For this review, take the finished solid that the model builds, in its own axes (mm). Round coordinates to 2 decimals unless told otherwise and drop trailing zeros. Loops run counter-clockwise (first coordinate to the right, second up) from the corner with the lowest first, then second, coordinate; pieces in that order, holes last. Notation, with made-up numbers: (34, 15.5) -> (88, 15.5) arc R10 cw to (88, 34.5) -> close; hole circle Ø11 at (10, 19). An arc over 180 degrees is marked (long way). Use one line per item in the form item = value. Start each with the question number.
from build123d import *

# Parameters (mm, degrees)
SKETCH_1_R          = 1.25
SKETCH_1_R_2        = 6.55
EXTRUDE_1_DEPTH     = 1.5
EXTRUDE_2_DEPTH     = 3
SKETCH_3_R          = 0.6
CUT_EXTRUDE_1_DEPTH = 4
SKETCH_4_R          = 1.55
CUT_EXTRUDE_2_DEPTH = 4
CUT_EXTRUDE_3_DEPTH = 4
FILLET_1_R          = 1
CHAMFER_1_SIZE      = 1
SKETCH_6_R          = 1.55
EXTRUDE_3_DEPTH     = 3
CUT_EXTRUDE_4_DEPTH = 4
FILLET_2_R          = 0.6


with BuildPart() as part:
    # 草图1 → 凸台-拉伸1 (new body, symmetric)
    with BuildSketch(Plane.XY):
        with BuildLine():
            Line((-34.52642222, 8.609923977), (-26.496675247, -8.609923977))
            Line((-26.496675247, -8.609923977), (26.496675247, -8.609923977))
            Line((26.496675247, -8.609923977), (34.52642222, 8.609923977))
            Line((34.52642222, 8.609923977), (5.071419141, 22.345017483))
            ThreePointArc((5.071419141, 22.345017483), (0, 23.469324039), (-5.071419141, 22.345017483))
            Line((-5.071419141, 22.345017483), (-34.52642222, 8.609923977))
        make_face()
        with Locations((0, 20.969324039)):
            Circle(SKETCH_1_R, mode=Mode.SUBTRACT)
        with Locations((8.227241336, 6.719324039)):
            Circle(SKETCH_1_R, mode=Mode.SUBTRACT)
        with Locations((-8.227241336, 6.719324039)):
            Circle(SKETCH_1_R, mode=Mode.SUBTRACT)
        with Locations((0, 11.469324039)):
            Circle(SKETCH_1_R_2, mode=Mode.SUBTRACT)
    extrude(amount=EXTRUDE_1_DEPTH, both=True)

    # 草图2 → 凸台-拉伸2 (add)
    with BuildSketch(Plane.XY.offset(1.5)):
        Polygon((-33.258567434, 5.891000616), (-38.696414157, 3.355291045), (-33.202376754, -8.426710186), (-27.764530032, -5.891000616), (-29.032384817, -3.172077255), (-31.705992789, -4.418801127), (-34.664320621, 1.925353382), (-31.990712649, 3.172077255), align=None)
        Polygon((38.696414157, 3.355291045), (33.202376754, -8.426710186), (27.764530032, -5.891000616), (29.032384817, -3.172077255), (31.705992789, -4.418801127), (34.664320621, 1.925353382), (31.990712649, 3.172077255), (33.258567434, 5.891000616), align=None)
    extrude(amount=-EXTRUDE_2_DEPTH)

    # 草图3 → 切除-拉伸1 (cut, through all)
    with BuildSketch(Plane.XY.offset(1.5)):
        with Locations((-33.512138391, 6.434785288)):
            Circle(SKETCH_3_R)
        with Locations((-34.410749664, 1.38156871)):
            Circle(SKETCH_3_R)
        with Locations((-31.959563746, -3.875016455)):
            Circle(SKETCH_3_R)
        with Locations((-29.285955774, -2.628292582)):
            Circle(SKETCH_3_R)
        with Locations((-31.737141692, 2.628292582)):
            Circle(SKETCH_3_R)
        with Locations((-27.510959075, -6.434785288)):
            Circle(SKETCH_3_R)
        with Locations((27.510959075, -6.434785288)):
            Circle(SKETCH_3_R)
        with Locations((31.737141692, 2.628292582)):
            Circle(SKETCH_3_R)
        with Locations((29.285955774, -2.628292582)):
            Circle(SKETCH_3_R)
        with Locations((31.959563746, -3.875016455)):
            Circle(SKETCH_3_R)
        with Locations((34.410749664, 1.38156871)):
            Circle(SKETCH_3_R)
        with Locations((33.512138391, 6.434785288)):
            Circle(SKETCH_3_R)
    extrude(amount=-CUT_EXTRUDE_1_DEPTH, mode=Mode.SUBTRACT)

    # 草图4 → 切除-拉伸2 (cut, through all)
    with BuildSketch(Plane.XY.offset(1.5)):
        with Locations((-29.875181049, 6.917010638)):
            Circle(SKETCH_4_R)
        with Locations((-24.803761908, -3.958682806)):
            Circle(SKETCH_4_R)
        with Locations((24.803761908, -3.958682806)):
            Circle(SKETCH_4_R)
        with Locations((29.875181049, 6.917010638)):
            Circle(SKETCH_4_R)
    extrude(amount=-CUT_EXTRUDE_2_DEPTH, mode=Mode.SUBTRACT)

    # 草图5 → 切除-拉伸3 (cut, through all)
    with BuildSketch(Plane.XY.offset(1.5)):
        with BuildLine():
            Line((-11.487209375, 14.939773688), (-26.491794663, 7.943020661))
            Line((-26.491794663, 7.943020661), (-21.50545883, -2.750211042))
            Line((-21.50545883, -2.750211042), (-10.562941581, 5.775093172))
            ThreePointArc((-10.562941581, 5.775093172), (-11.939435981, 10.265219199), (-11.487209375, 14.939773688))
        make_face()
        with BuildLine():
            Line((-17.384057406, -4.609923977), (-2, -4.609923977))
            Line((-2, -4.609923977), (-2, -0.362835527))
            ThreePointArc((-2, -0.362835527), (-5.267782675, 0.687373117), (-8.104582376, 2.619705713))
            Line((-8.104582376, 2.619705713), (-17.384057406, -4.609923977))
        make_face()
        with BuildLine():
            Line((17.384057406, -4.609923977), (8.104582376, 2.619705713))
            ThreePointArc((8.104582376, 2.619705713), (5.267782675, 0.687373117), (2, -0.362835527))
            Line((2, -0.362835527), (2, -4.609923977))
            Line((2, -4.609923977), (17.384057406, -4.609923977))
        make_face()
        with BuildLine():
            Line((21.50545883, -2.750211042), (10.562941581, 5.775093172))
            ThreePointArc((10.562941581, 5.775093172), (11.939435981, 10.265219199), (11.487209375, 14.939773688))
            Line((11.487209375, 14.939773688), (26.491794663, 7.943020661))
            Line((26.491794663, 7.943020661), (21.50545883, -2.750211042))
        make_face()
    extrude(amount=-CUT_EXTRUDE_3_DEPTH, mode=Mode.SUBTRACT)

    # 圆角1
    fillet_1_edges = [part.edges().sort_by_distance(p)[0] for p in [
        (-2, -0.362835527, 0),
        (-2, -4.609923977, 0),
        (-17.384057406, -4.609923977, 0),
        (-8.104582376, 2.619705713, 0),
        (17.384057406, -4.609923977, 0),
        (2, -4.609923977, 0),
        (2, -0.362835527, 0),
        (8.104582376, 2.619705713, 0),
        (10.562941581, 5.775093172, 0),
        (11.487209375, 14.939773688, 0),
        (26.491794663, 7.943020661, 0),
        (21.50545883, -2.750211042, 0),
        (-21.50545883, -2.750211042, 0),
        (-26.491794663, 7.943020661, 0),
        (-11.487209375, 14.939773688, 0),
        (-10.562941581, 5.775093172, 0),
    ]]
    fillet(fillet_1_edges, radius=FILLET_1_R)

    # 倒角1
    chamfer_1_edges = [part.edges().sort_by_distance(p)[0] for p in [
        (-33.202376754, -8.426710186, 0),
        (-38.696414157, 3.355291045, 0),
        (38.696414157, 3.355291045, 0),
        (33.202376754, -8.426710186, 0),
    ]]
    chamfer(chamfer_1_edges, length=CHAMFER_1_SIZE)

    # 草图6 → 凸台-拉伸3 (add)
    with BuildSketch(Plane.XY.offset(1.5)):
        with BuildLine():
            Line((-11.457456133, 28.190053348), (-20.630385749, 15.089752201))
            Line((-20.630385749, 15.089752201), (-5.071419141, 22.345017483))
            ThreePointArc((-5.071419141, 22.345017483), (0, 23.469324039), (5.071419141, 22.345017483))
            Line((5.071419141, 22.345017483), (20.630385749, 15.089752201))
            Line((20.630385749, 15.089752201), (11.457456133, 28.190053348))
            ThreePointArc((11.457456133, 28.190053348), (10.38524584, 29.130356539), (9, 29.469324039))
            Line((9, 29.469324039), (-9, 29.469324039))
            ThreePointArc((-9, 29.469324039), (-10.38524584, 29.130356539), (-11.457456133, 28.190053348))
        make_face()
        with Locations((-9, 26.469324039)):
            Circle(SKETCH_6_R, mode=Mode.SUBTRACT)
        with Locations((9, 26.469324039)):
            Circle(SKETCH_6_R, mode=Mode.SUBTRACT)
    extrude(amount=-EXTRUDE_3_DEPTH)

    # 草图7 → 切除-拉伸4 (cut, through all)
    with BuildSketch(Plane.XY.offset(1.5)):
        with BuildLine():
            Line((-9.803167106, 23.578835741), (-13.379923452, 18.470698295))
            Line((-13.379923452, 18.470698295), (-9.745807228, 18.470698295))
            ThreePointArc((-9.745807228, 18.470698295), (0, 23.469324039), (9.745807228, 18.470698295))
            Line((9.745807228, 18.470698295), (13.379923452, 18.470698295))
            Line((13.379923452, 18.470698295), (9.803167106, 23.578835741))
            ThreePointArc((9.803167106, 23.578835741), (7.422496962, 23.917563046), (6.055342113, 25.895747603))
            Line((6.055342113, 25.895747603), (-6.055342113, 25.895747603))
            ThreePointArc((-6.055342113, 25.895747603), (-7.422496962, 23.917563046), (-9.803167106, 23.578835741))
        make_face()
    extrude(amount=-CUT_EXTRUDE_4_DEPTH, mode=Mode.SUBTRACT)

    # 圆角2
    fillet_2_edges = [part.edges().sort_by_distance(p)[0] for p in [
        (-9.803167106, 23.578835741, 0),
        (-6.055342113, 25.895747603, 0),
        (6.055342113, 25.895747603, 0),
        (9.803167106, 23.578835741, 0),
        (13.379923452, 18.470698295, 0),
        (9.745807228, 18.470698295, 0),
        (-9.745807228, 18.470698295, 0),
        (-13.379923452, 18.470698295, 0),
    ]]
    fillet(fillet_2_edges, radius=FILLET_2_R)


solid = part.part
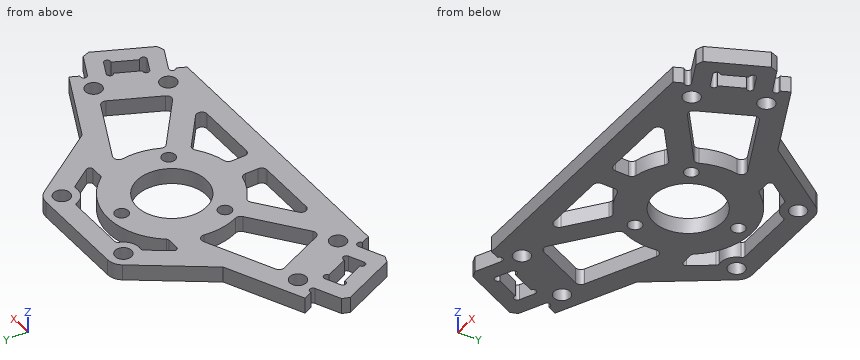
Item 1: Wall thickness on line 1 (Y direction, x = -29.5, z = 0.65); line 2 (X direction, y = 4, z = -0.55); line 3 (Y direction, x = 13.5, z = 0.8): over which ranges is each line inside the solid? List them lowest first.
Item 2: Take a section at A-A on x = 0. Give the boundary of the cut face in (y, z), plus the area to 3 significant figures.
Item 3: Take a section at B-B on x = -19. Give the boundary of the cut face in (y, z), plus the area to 3 significant figures.
Item 4: For P1, Ø1.1, axis at x = -11, z = -0.5, coming from the +Y side; P2, Ø5, axis at x = -9, y = 26.47, coming from the +Z side, all flat-tipped, find the tip position at first contact; note any pin that passes through.
Item 5: Take a section at C-C on z = 0.35. Give the number of separate pieces and of enclosed holes in the cut face, plus the area to 3 significant figures.
Results:
q1.line_1 = -6.7 to -3.39, -2.07 to 5.41, 8.42 to 10.95
q1.line_2 = -37.31 to -24.65, -12.84 to 12.84, 24.65 to 37.31
q1.line_3 = -8.61 to -4.61, -1.58 to 3.49, 14 to 25.27
q2.outline = (-8.61, -1.5) -> (4.92, -1.5) -> (4.92, 1.5) -> (-8.61, 1.5) -> close; (18.02, -1.5) -> (19.72, -1.5) -> (19.72, 1.5) -> (18.02, 1.5) -> close; (22.22, -1.5) -> (23.47, -1.5) -> (23.47, 1.5) -> (22.22, 1.5) -> close; (25.9, -1.5) -> (29.47, -1.5) -> (29.47, 1.5) -> (25.9, 1.5) -> close
q2.area = 60.2 mm2
q3.outline = (-8.61, -1.5) -> (-0.8, -1.5) -> (-0.8, 1.5) -> (-8.61, 1.5) -> close; (11.44, -1.5) -> (17.42, -1.5) -> (17.42, 1.5) -> (11.44, 1.5) -> close
q3.area = 41.4 mm2
q4.P1 = 29.1
q4.P2 = 1.5
q5.separate_pieces = 1
q5.enclosed_holes = 17
q5.area = 1,270 mm2
